Part print with two shaded views. Sizes in mm from the minimum x, y, z corner. A direction names the side the tool comes from. Give positions to 0.01 mm unless a question says otherwise; leave off trailing zeros. Write each loop counter-clockwise with the first axis right and the second up, starting at its lowest first coordinate (ties: lowest second). Pieces come first, ordered by that corner, then holes. Notation, with made-up numbers: M 37.5,24.5 L 93.5,24.5 A30 cw 93.5,48.5 Z; hole C 2,-10 d7. An arc over 180 degrees is marked long. One line per item, written item: value. Start each with the question number.
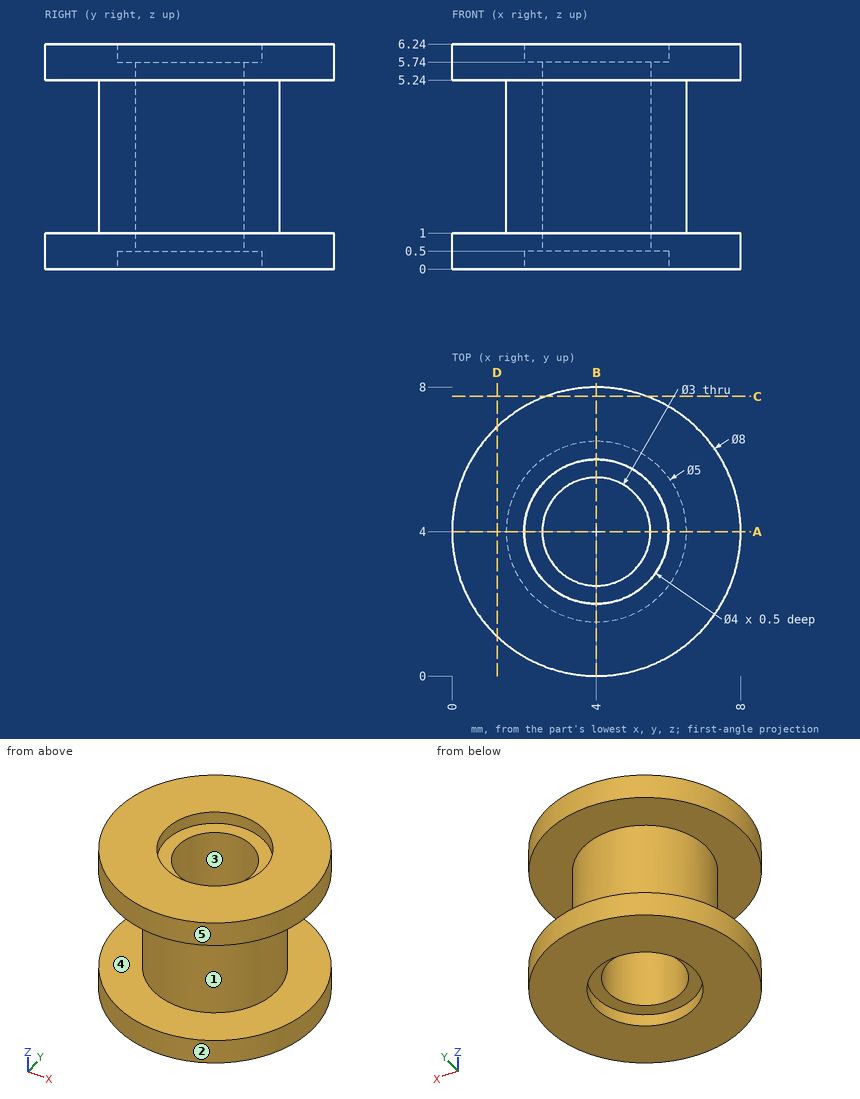
1) Drop flat-ended pins along their axis: P1, Ø1.5, axis at y = 6, z = 5.5, coming from the +X side; P2, Ø3, axis at y = 4.5, z = 1.5, coming from the +X side; P3, Ø3.5, axis at x = 4, y = 4, coming from the -Z side; P4, Ø3, axis at x = 3.5, z = 3.5, coming from the +Y side. Give the stop position or say it passes through.
2) Tool access for the marked faces 1 and 2: list every direction of +Z, -Z, +X, -X, +Y, -Y with a clear straight run to the whole face (end or side of a thin tool).
3) Band-saw the part on D-D (x = 1.25). List the corners of the cut face in (y, z), then the cut area to 3 significant figures.
4) Band-saw the part on A-A (y = 4). List the corners of the cut face in (x, z), then the cut area to 3 significant figures.
5) Mould opens along Y. For the marked faces 3, 4 and 5 say: released by +Y, released by -Y, zero draft, split by the parting line, or undercut.
6) Band-saw the part on C-C (y = 7.75). List the corners of the cut face in (x, z).
7) Probe line 1 along Z through (x, y) = (4.5, 0.75); line 2 along Y through (x, z) = (4, 1.7); line 3 along Y through (x, z) = (4, 5.9). List the from-to ranges inside material, lowest first. Write a range as from..to.
Model answer:
1. P1: stops at x = 7.8
1. P2: stops at x = 8
1. P3: stops at z = 0.5
1. P4: stops at y = 6.5
2. face 1: none
2. face 2: +Z, -Z
3. outline: M 1.1,0 L 6.9,0 L 6.9,1 L 1.1,1 Z; M 1.1,5.24 L 6.9,5.24 L 6.9,6.24 L 1.1,6.24 Z
3. area: 11.6 mm²
4. outline: M 0,0 L 2,0 L 2,0.5 L 2.5,0.5 L 2.5,5.74 L 2,5.74 L 2,6.24 L 0,6.24 L 0,5.24 L 1.5,5.24 L 1.5,1 L 0,1 Z; M 5.5,0.5 L 6,0.5 L 6,0 L 8,0 L 8,1 L 6.5,1 L 6.5,5.24 L 8,5.24 L 8,6.24 L 6,6.24 L 6,5.74 L 5.5,5.74 Z
4. area: 17.5 mm²
5. face 3: undercut
5. face 4: zero draft
5. face 5: split by the parting line
6. outline: M 2.61,0 L 5.39,0 L 5.39,1 L 2.61,1 Z; M 2.61,5.24 L 5.39,5.24 L 5.39,6.24 L 2.61,6.24 Z
7. line 1: z = 0..1, 5.24..6.24
7. line 2: y = 1.5..2.5, 5.5..6.5
7. line 3: y = 0..2, 6..8
